Check sheet for the modelled part. Datum: model origin and axes. Units: mm. A direction names the side the tool comes from. Coordinates: 2 decimals unless noted, no trailing zeros. Loops run counter-clockwise (first coordinate to the right, second up) from the corner with the lowest first, then second, coordinate; pieces in that order, holes last. Notation, with made-up numbers: (-33.5, 23) - (-0.5, 23) arc R22 ccw to (-0.5, 55) - close; hole circle Ø10 at (57.5, 78.25). An arc over 180 degrees is marked (long way). Use a Markdown table: item, result. Add a question column.
1) Thickness scan on line 1 (Z direction, x = 26.5, y = 20); line 2 (X direction, y = 27, z = 11.5); line 3 (Z direction, x = 15, y = 9). Record the ranges inside material, lowest first.
2) Sectioned sample at C-C, the plane x = 21. Enter the section's corners in (y, z).
3) Sectioned sample at D-D, the plane z = 20. Enter the section's corners in (x, y), then the cut area to 3 significant figures.
4) Tool access check on faces 1 (the flat face through (17, 25, 23)), 2 (the cylindrical face through (17.6, 32.43, 22.75)), 3 (the flat face through (25, 25, 38)). Record the directions out of +Z, -Z, +X, -X, +Y, -Y that give a thin tool (end or side, any length) a straight path to the whole face; none if there is none.
5) Sectioned sample at A-A, the plane z = 34. Enter the section's corners in (x, y).
6) Go/stop test with flat-tipped pins: P1, Ø8, axis at y = 27, z = 33, coming from the -X side; P2, Ø10, axis at y = 18.5, z = 30, coming from the +X side; P3, Ø3, axis at x = 10, y = 43, coming from the +Z side; P4, Ø10, axis at x = 22.5, y = 27.5, coming from the -Z side. Record where each tip stops, or that it passes through.
7) Sectioned sample at B-B, the plane y = 20. Enter the section's corners in (x, z), then the cut area to 3 significant figures.
from build123d import *

# Parameters (mm, degrees)
F0_W         = 50
F0_H         = 50
F1_DEPTH     = 3
F2_W         = 16
F2_H         = 16
F3_DEPTH     = 40
F4_W         = 12.2
F4_H         = 10.2
F5_DEPTH     = 16
F6_T1_DEPTH  = 12
F6_T3_DEPTH  = 12
F6_T5_DEPTH  = 38
F6_S9_W      = 2
F6_S9_H      = 2
F6_T10_DEPTH = 2
F6_S15_W     = 2
F6_S15_H     = 2
F6_T16_DEPTH = 2
F6_S21_W     = 2
F6_S21_H     = 2
F6_T22_DEPTH = 2
F6_S27_W     = 2
F6_S27_H     = 2
F6_T28_DEPTH = 2
F6_T31_DEPTH = 12
F6_T33_DEPTH = 12
F6_T36_ANGLE = 90
F6_T38_ANGLE = 90
F6_T40_ANGLE = 90
F6_T42_ANGLE = 90
F7_R         = 5


# Not quite as in the source:
# - a fillet or chamfer that OpenCascade refuses, or shapes differently, is made with other operations: its cross-section is extruded or revolved along the edge and cut away or added


with BuildPart() as f1:
    # F0 (on Top) → F1 (new body)
    with BuildSketch(Plane.XY):
        with Locations((25, 25)):
            Rectangle(F0_W, F0_H)
    extrude(amount=F1_DEPTH)

    # F2 (on face) → F3 (join)
    with BuildSketch(Plane.XY.offset(3)):
        with Locations((25, 25)):
            Rectangle(F2_W, F2_H)
    extrude(amount=F3_DEPTH)

    # F4 (on face) → F5 (cut)
    with BuildSketch(Plane.XZ.offset(-17)):
        with Locations((25, 32.9)):
            Rectangle(F4_W, F4_H)
    extrude(amount=-F5_DEPTH, mode=Mode.SUBTRACT)

    # F6: fillet of radius 2 on 12 edges, made by hand

    # F6_s2 → F6_t1 (cut)
    with BuildSketch(Plane.YZ.offset(19)):
        with BuildLine():
            ThreePointArc((17, 41), (17.5857864376, 42.4142135624), (19, 43))
            Line((19, 43), (17, 43))
            Line((17, 43), (17, 41))
        make_face()
        with BuildLine():
            ThreePointArc((33, 41), (32.4142135624, 42.4142135624), (31, 43))
            Line((31, 43), (33, 43))
            Line((33, 43), (33, 41))
        make_face()
    extrude(amount=F6_T1_DEPTH, mode=Mode.SUBTRACT)

    # F6_s4 → F6_t3 (cut)
    with BuildSketch(Plane.XZ.offset(-31)):
        with BuildLine():
            ThreePointArc((33, 41), (32.4142135624, 42.4142135624), (31, 43))
            Line((31, 43), (33, 43))
            Line((33, 43), (33, 41))
        make_face()
        with BuildLine():
            ThreePointArc((17, 41), (17.5857864376, 42.4142135624), (19, 43))
            Line((19, 43), (17, 43))
            Line((17, 43), (17, 41))
        make_face()
    extrude(amount=F6_T3_DEPTH, mode=Mode.SUBTRACT)

    # F6_s6 → F6_t5 (cut)
    with BuildSketch(Plane.XY.offset(3)):
        with BuildLine():
            ThreePointArc((31, 17), (32.4142135624, 17.5857864376), (33, 19))
            Line((33, 19), (33, 17))
            Line((33, 17), (31, 17))
        make_face()
        with BuildLine():
            ThreePointArc((31, 33), (32.4142135624, 32.4142135624), (33, 31))
            Line((33, 31), (33, 33))
            Line((33, 33), (31, 33))
        make_face()
        with BuildLine():
            ThreePointArc((17, 19), (17.5857864376, 17.5857864376), (19, 17))
            Line((19, 17), (17, 17))
            Line((17, 17), (17, 19))
        make_face()
        with BuildLine():
            ThreePointArc((19, 33), (17.5857864376, 32.4142135624), (17, 31))
            Line((17, 31), (17, 33))
            Line((17, 33), (19, 33))
        make_face()
    extrude(amount=F6_T5_DEPTH, mode=Mode.SUBTRACT)


with BuildPart() as f6_tool8:
    # F6_s9 → F6_t10 (new body)
    with BuildSketch(Plane.XZ.offset(-19)):
        with Locations((18, 42)):
            Rectangle(F6_S9_W, F6_S9_H)
    extrude(amount=F6_T10_DEPTH)

    # F6_s11 → F6_t12 (revolve, cut)
    with BuildSketch(Plane(origin=(19, 19, 41), x_dir=(0.7071067812, 0, -0.7071067812), z_dir=(-0.7071067812, 0, -0.7071067812))):
        with BuildLine():
            ThreePointArc((0, -2), (2, 0), (0, 2))
            Line((0, 2), (0, -2))
        make_face()
    revolve(axis=Axis((19, 19, 41), (0, -1, 0)), mode=Mode.SUBTRACT)


with BuildPart() as f1_1:
    add(f1.part)

    # F6_t7: cut F6_tool8
    add(f6_tool8.part, mode=Mode.SUBTRACT)


with BuildPart() as f6_tool14:
    # F6_s15 → F6_t16 (new body)
    with BuildSketch(Plane.XZ.offset(-19)):
        with Locations((32, 42)):
            Rectangle(F6_S15_W, F6_S15_H)
    extrude(amount=F6_T16_DEPTH)

    # F6_s17 → F6_t18 (revolve, cut)
    with BuildSketch(Plane(origin=(31, 19, 41), x_dir=(-0.7071067812, 0, -0.7071067812), z_dir=(-0.7071067812, 0, 0.7071067812))):
        with BuildLine():
            ThreePointArc((0, -2), (2, 0), (0, 2))
            Line((0, 2), (0, -2))
        make_face()
    revolve(axis=Axis((31, 19, 41), (0, -1, 0)), mode=Mode.SUBTRACT)


with BuildPart() as f1_2:
    add(f1_1.part)

    # F6_t13: cut F6_tool14
    add(f6_tool14.part, mode=Mode.SUBTRACT)


with BuildPart() as f6_tool20:
    # F6_s21 → F6_t22 (new body)
    with BuildSketch(Plane.YZ.offset(31)):
        with Locations((32, 42)):
            Rectangle(F6_S21_W, F6_S21_H)
    extrude(amount=F6_T22_DEPTH)

    # F6_s23 → F6_t24 (revolve, cut)
    with BuildSketch(Plane(origin=(31, 31, 41), x_dir=(0, -0.7071067812, -0.7071067812), z_dir=(0, -0.7071067812, 0.7071067812))):
        with BuildLine():
            ThreePointArc((0, -2), (2, 0), (0, 2))
            Line((0, 2), (0, -2))
        make_face()
    revolve(axis=Axis((31, 31, 41), (1, 0, 0)), mode=Mode.SUBTRACT)


with BuildPart() as f1_3:
    add(f1_2.part)

    # F6_t19: cut F6_tool20
    add(f6_tool20.part, mode=Mode.SUBTRACT)


with BuildPart() as f6_tool26:
    # F6_s27 → F6_t28 (new body)
    with BuildSketch(Plane.XY.offset(41)):
        with Locations((18, 32)):
            Rectangle(F6_S27_W, F6_S27_H)
    extrude(amount=F6_T28_DEPTH)

    # F6_s29 → F6_t30 (revolve, cut)
    with BuildSketch(Plane(origin=(19, 31, 41), x_dir=(0.7071067812, -0.7071067812, 0), z_dir=(-0.7071067812, -0.7071067812, 0))):
        with BuildLine():
            ThreePointArc((0, -2), (2, 0), (0, 2))
            Line((0, 2), (0, -2))
        make_face()
    revolve(axis=Axis((19, 31, 41), (0, 0, 1)), mode=Mode.SUBTRACT)


with BuildPart() as f1_4:
    add(f1_3.part)

    # F6_t25: cut F6_tool26
    add(f6_tool26.part, mode=Mode.SUBTRACT)

    # F6_s32 → F6_t31 (join)
    with BuildSketch(Plane.YZ.offset(19)):
        with BuildLine():
            ThreePointArc((15, 3), (16.4142135624, 3.5857864376), (17, 5))
            Line((17, 5), (17, 3))
            Line((17, 3), (15, 3))
        make_face()
        with BuildLine():
            ThreePointArc((35, 3), (33.5857864376, 3.5857864376), (33, 5))
            Line((33, 5), (33, 3))
            Line((33, 3), (35, 3))
        make_face()
    extrude(amount=F6_T31_DEPTH)

    # F6_s34 → F6_t33 (join)
    with BuildSketch(Plane.XZ.offset(-31)):
        with BuildLine():
            ThreePointArc((35, 3), (33.5857864376, 3.5857864376), (33, 5))
            Line((33, 5), (33, 3))
            Line((33, 3), (35, 3))
        make_face()
        with BuildLine():
            ThreePointArc((15, 3), (16.4142135624, 3.5857864376), (17, 5))
            Line((17, 5), (17, 3))
            Line((17, 3), (15, 3))
        make_face()
    extrude(amount=F6_T33_DEPTH)

    # F6_s35 → F6_t36 (revolve)
    with BuildSketch(Plane.YZ.offset(31)):
        with BuildLine():
            ThreePointArc((35, 3), (33.5857864376, 3.5857864376), (33, 5))
            Line((33, 5), (33, 3))
            Line((33, 3), (35, 3))
        make_face()
    revolve(axis=Axis((31, 31, 3), (0, 0, -1)), revolution_arc=F6_T36_ANGLE)

    # F6_s37 → F6_t38 (revolve)
    with BuildSketch(Plane.YZ.offset(19)):
        with BuildLine():
            ThreePointArc((35, 3), (33.5857864376, 3.5857864376), (33, 5))
            Line((33, 5), (33, 3))
            Line((33, 3), (35, 3))
        make_face()
    revolve(axis=Axis((19, 31, 3), (0, 0, 1)), revolution_arc=F6_T38_ANGLE)

    # F6_s39 → F6_t40 (revolve)
    with BuildSketch(Plane.XZ.offset(-19)):
        with BuildLine():
            ThreePointArc((15, 3), (16.4142135624, 3.5857864376), (17, 5))
            Line((17, 5), (17, 3))
            Line((17, 3), (15, 3))
        make_face()
    revolve(axis=Axis((19, 19, 3), (0, 0, 1)), revolution_arc=F6_T40_ANGLE)

    # F6_s41 → F6_t42 (revolve)
    with BuildSketch(Plane.YZ.offset(31)):
        with BuildLine():
            ThreePointArc((15, 3), (16.4142135624, 3.5857864376), (17, 5))
            Line((17, 5), (17, 3))
            Line((17, 3), (15, 3))
        make_face()
    revolve(axis=Axis((31, 19, 3), (0, 0, 1)), revolution_arc=F6_T42_ANGLE)

    # F7
    f7_edges = [f1_4.edges().sort_by_distance(p)[0] for p in [
        (0, 0, 1.5),
        (50, 0, 1.5),
        (0, 50, 1.5),
        (50, 50, 1.5),
    ]]
    fillet(f7_edges, radius=F7_R)


solid = f1_4.part
Solved:
| question | item | result |
|---|---|---|
| 1 | line 1 | z = 0 to 27.8, 38 to 43 |
| 1 | line 2 | x = 17 to 33 |
| 1 | line 3 | z = 0 to 3 |
| 2 | outline | (0, 0) - (50, 0) - (50, 3) - (35, 3) arc R2 cw to (33, 5) - (33, 27.8) - (17, 27.8) - (17, 5) arc R2 cw to (15, 3) - (0, 3) - close; (17, 38) - (33, 38) - (33, 41) arc R2 ccw to (31, 43) - (19, 43) arc R2 ccw to (17, 41) - close |
| 3 | outline | (17, 19) arc R2 ccw to (19, 17) - (31, 17) arc R2 ccw to (33, 19) - (33, 31) arc R2 ccw to (31, 33) - (19, 33) arc R2 ccw to (17, 31) - close |
| 3 | area | 253 mm2 |
| 4 | face 1 | +Z, -X, +Y, -Y |
| 4 | face 2 | +Z, -X, +Y |
| 4 | face 3 | +Y, -Y |
| 5 | outline | (17, 19) arc R2 ccw to (18.9, 17) - (18.9, 33) arc R2 ccw to (17, 31) - close; (31.1, 17) arc R2 ccw to (33, 19) - (33, 31) arc R2 ccw to (31.1, 33) - close |
| 6 | P1 | stops at x = 17 |
| 6 | P2 | stops at x = 33 |
| 6 | P3 | stops at z = 3 |
| 6 | P4 | stops at z = 0 |
| 7 | outline | (0, 0) - (50, 0) - (50, 3) - (35, 3) arc R2 cw to (33, 5) - (33, 41) arc R2 ccw to (31, 43) - (19, 43) arc R2 ccw to (17, 41) - (17, 5) arc R2 cw to (15, 3) - (0, 3) - close; hole (18.9, 27.8) - (31.1, 27.8) - (31.1, 38) - (18.9, 38) - close |
| 7 | area | 666 mm2 |
